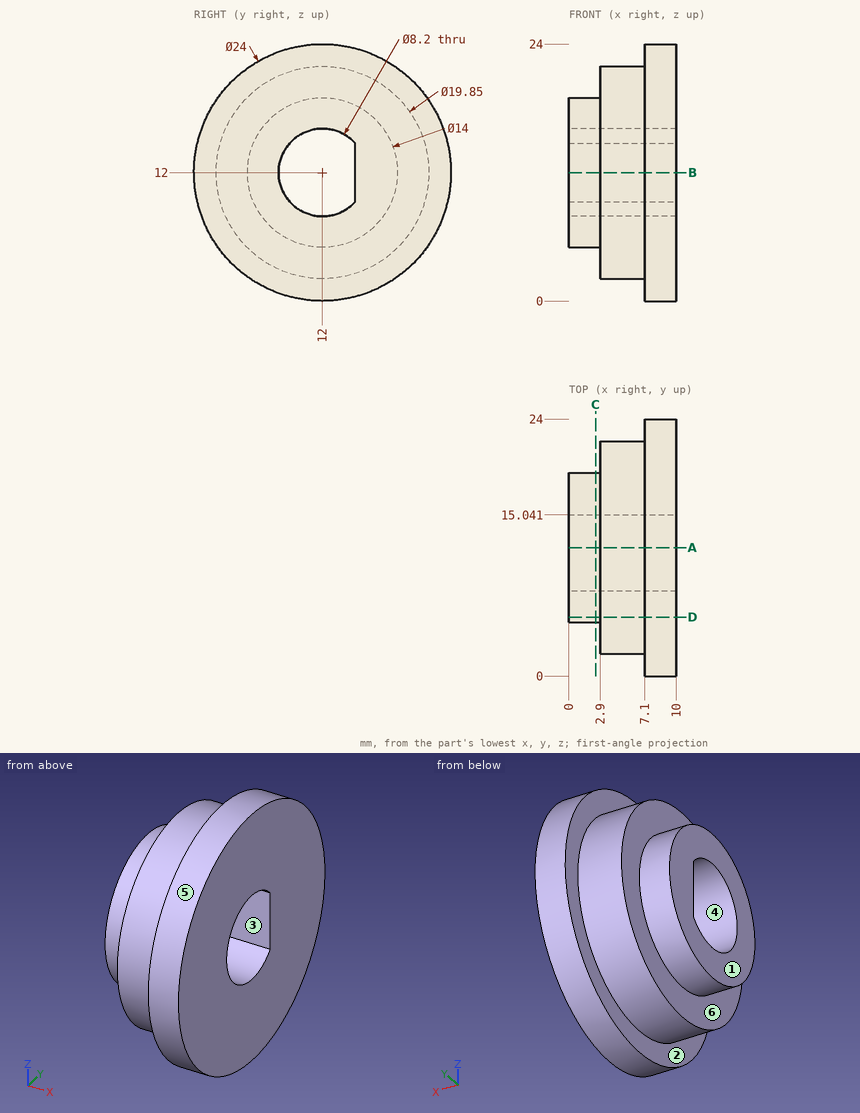
Here's the drawing with two shaded views (mm, measured from the low corner). I have some questions. A direction names the side the tool comes from. Give positions to 0.01 mm unless a question says otherwise; leave off trailing zeros. Loops run counter-clockwise (first coordinate to the right, second up) from the corner with the lowest first, then second, coordinate; pieces in that order, holes last. Notation, with made-up numbers: M 26.25,-5.5 L 82.25,-5.5 A18 ccw 82.25,14.5 Z; hole C 51,15 d4. An arc over 180 degrees is marked long. Use one line per item in the form item = value. Start each with the question number.
(1) I want a section at C-C, the plane x = 2.5. Write out the boundary of the cut face in (y, z).
(2) Thinking about a two-plate mould opening in Z: for the marked faces 4, 5 and 6, which applies, released by +Z, released by -Z, zero draft, split by the parting line, or undercut?
(3) I want a section at B-B, the plane z = 12. Write out the boundary of the cut face in (x, y) (3 decimals).
(4) I want a section at D-D, the plane y = 5.5. Write out the boundary of the cut face in (x, z).
(5) I'm going to push flat-ended pins straight in: P1, Ø6, axis at x = 8.5, y = 18, coming from the -Z side; P2, Ø1.5, axis at x = 8, y = 14.5, coming from the +Z side; P3, Ø1, axis at x = 7, z = 11, coming from the +Y side. Where does each tip first touch, or does it pass through?
(6) I want a section at A-A, the plane y = 12. Write out the boundary of the cut face in (x, z) (3 decimals).
(7) Please list where these lines run through material, in increasing order: line 1 (Y direction, x = 3, z = 12) (3 decimals); line 2 (Y direction, x = 8, z = 12); line 3 (X direction, y = 20.25, z = 9.25).
(8) On a 3-axis mill with a long thin cutter (end or side, diameter ignored), from which of +Z, -Z, +X, -X, +Y, -Y can I reach the whole of each face in a straight line? I mean the marked faces 1, 2 and 3. Say none if no direction works.
Worked out:
q1.outline = C 12,12 d14; hole M 15.04,9.25 L 15.04,14.75 A4.1 ccw long Z
q2.face_4 = undercut
q2.face_5 = split by the parting line
q2.face_6 = zero draft
q3.outline = M 0,5 L 2.9,5 L 2.9,2.075 L 7.1,2.075 L 7.1,0 L 10,0 L 10,7.9 L 0,7.9 Z; M 0,15.041 L 10,15.041 L 10,24 L 7.1,24 L 7.1,21.925 L 2.9,21.925 L 2.9,19 L 0,19 Z
q4.outline = M 0,9.4 L 2.9,9.4 L 2.9,4.5 L 7.1,4.5 L 7.1,1.91 L 10,1.91 L 10,22.09 L 7.1,22.09 L 7.1,19.5 L 2.9,19.5 L 2.9,14.6 L 0,14.6 Z
q5.P1 = 0.38
q5.P2 = 23.87
q5.P3 = 23.99
q6.outline = M 0,5 L 2.9,5 L 2.9,2.075 L 7.1,2.075 L 7.1,0 L 10,0 L 10,7.9 L 0,7.9 Z; M 0,16.1 L 10,16.1 L 10,24 L 7.1,24 L 7.1,21.925 L 2.9,21.925 L 2.9,19 L 0,19 Z
q7.line_1 = 2.075 to 7.9, 15.041 to 21.925
q7.line_2 = 0 to 7.9, 15.04 to 24
q7.line_3 = 2.9 to 10
q8.face_1 = +Z, -Z, -X, +Y, -Y
q8.face_2 = -X
q8.face_3 = +X, -X
